Part model, mm, in its own coordinate system. A direction names the side the tool comes from. Round coordinates to 2 decimals unless told otherwise and drop trailing zeros. Order: outer loops, then holes, each group sorted by start corner. A loop starts at its lowest first (then second) coordinate and runs counter-clockwise, first axis right, second up. Notation, with made-up numbers: (73.25, 78.5) - (94.25, 78.5) arc R30 cw to (94.25, 101.5) - close; hole circle Ø7 at (87, 58.5). An arc over 180 degrees is marked (long way). Answer as a JSON object with one key per item and string values.
```python
from build123d import *

# Parameters (mm, degrees)
ESBO_O1_W                = 20
ESBO_O1_H                = 20
RESSALTO_EXTRUS_O1_DEPTH = 20
ESBO_O2_R                = 5
RESSALTO_EXTRUS_O2_DEPTH = 12
ESBO_O3_R                = 5
RESSALTO_EXTRUS_O3_DEPTH = 12
RESSALTO_EXTRUS_O4_START = 12
ESBO_O4_R                = 5
RESSALTO_EXTRUS_O4_DEPTH = 12
RESSALTO_EXTRUS_O5_START = 12
ESBO_O5_R                = 5
RESSALTO_EXTRUS_O5_DEPTH = 12
ESBO_O6_R                = 5
RESSALTO_EXTRUS_O6_DEPTH = 12
RESSALTO_EXTRUS_O7_START = 12
ESBO_O7_R                = 5
RESSALTO_EXTRUS_O7_DEPTH = 12


with BuildPart() as part:
    # Esboço1 → Ressalto-extrusão1 (new body)
    with BuildSketch(Plane.XY):
        Rectangle(ESBO_O1_W, ESBO_O1_H)
    extrude(amount=RESSALTO_EXTRUS_O1_DEPTH)

    # Esboço2 → Ressalto-extrusão2 (add)
    with BuildSketch(Plane(origin=(10, 0, 0), x_dir=(0, 0, -1), z_dir=(1, 0, 0))):
        with Locations((-10, 0)):
            Circle(ESBO_O2_R)
    extrude(amount=RESSALTO_EXTRUS_O2_DEPTH)

    # Esboço3 → Ressalto-extrusão3 (add)
    with BuildSketch(Plane(origin=(0, 10, 0), x_dir=(1, 0, 0), z_dir=(0, 1, 0))):
        with Locations(Location((0, -10, 0), (0, 0, 270))):
            Circle(ESBO_O3_R)
    extrude(amount=RESSALTO_EXTRUS_O3_DEPTH)

    # Esboço4 → Ressalto-extrusão4 (add)
    with BuildSketch(Plane.ZY.offset(10).offset(RESSALTO_EXTRUS_O4_START)):
        with Locations(Location((10, 0, 0), (0, 0, 180))):
            Circle(ESBO_O4_R)
    extrude(amount=-RESSALTO_EXTRUS_O4_DEPTH)

    # Esboço5 → Ressalto-extrusão5 (add)
    with BuildSketch(Plane.XZ.offset(10).offset(RESSALTO_EXTRUS_O5_START)):
        with Locations(Location((0, 10, 0), (0, 0, 90))):
            Circle(ESBO_O5_R)
    extrude(amount=-RESSALTO_EXTRUS_O5_DEPTH)

    # Esboço6 → Ressalto-extrusão6 (add)
    with BuildSketch(Plane(origin=(0, 0, 0), x_dir=(-1, 0, 0), z_dir=(0, 0, -1))):
        Circle(ESBO_O6_R)
    extrude(amount=RESSALTO_EXTRUS_O6_DEPTH)

    # Esboço7 → Ressalto-extrusão7 (add)
    with BuildSketch(Plane.XY.offset(20).offset(RESSALTO_EXTRUS_O7_START)):
        with Locations(Location((0, 0, 0), (0, 0, 180))):
            Circle(ESBO_O7_R)
    extrude(amount=-RESSALTO_EXTRUS_O7_DEPTH)


solid = part.part
```
Item 1: Drop flat-ended pins along their axis: P1, Ø3, axis at x = 8, z = 4.5, coming from the -Y side; P2, Ø1, axis at y = 3, z = 27, coming from the +X side; P3, Ø2, axis at y = -5, z = -1.5, coming from the +X side. Give the stop position or say it passes through.
Taken from the geometry:
{"P1": "y = -10", "P2": "x = 4.33", "P3": "x = 3"}
Item 2: Cut at D-D (y = -15). Write the cut outline in (x, z), plus the area to 3 significant figures.
Taken from the geometry:
{"outline": "circle Ø10 at (0, 10)", "area": "78.5 mm2"}
Item 3: Cut at A-A (z = 10). Write the cut outline in (x, y).
Taken from the geometry:
{"outline": "(-22, -5) - (-10, -5) - (-10, -10) - (-5, -10) - (-5, -22) - (5, -22) - (5, -10) - (10, -10) - (10, -5) - (22, -5) - (22, 5) - (10, 5) - (10, 10) - (5, 10) - (5, 22) - (-5, 22) - (-5, 10) - (-10, 10) - (-10, 5) - (-22, 5) - close"}
Item 4: Cut at B-B (y = 0). Write the cut outline in (x, z), plus the area to 3 significant figures.
Taken from the geometry:
{"outline": "(-22, 5) - (-10, 5) - (-10, 0) - (-5, 0) - (-5, -12) - (5, -12) - (5, 0) - (10, 0) - (10, 5) - (22, 5) - (22, 15) - (10, 15) - (10, 20) - (5, 20) - (5, 32) - (-5, 32) - (-5, 20) - (-10, 20) - (-10, 15) - (-22, 15) - close", "area": "880 mm2"}
Item 5: Probe L1, parallel to Z at x = -1, y = 7; L2, parallel to Y at x = -6, z = 10. List the from-to ranges inside material, lowest first. Write a range as from..to.
Taken from the geometry:
{"L1": "0..20", "L2": "-10..10"}
Item 6: Cut at C-C (x = -7). Write the cut outline in (y, z), plus the area to 3 significant figures.
Taken from the geometry:
{"outline": "(-10, 0) - (10, 0) - (10, 20) - (-10, 20) - close", "area": "400 mm2"}
Item 7: Tool access for faces 1 (the flat face through (10, -2, 5)), 2 (the flat face through (-2, -10, 5)), 3 (the cylindrical face through (1.08, -4.88, -5.92)): list every direction of +Z, -Z, +X, -X, +Y, -Y with a clear straight run to the whole face (end or side of a thin tool).
Taken from the geometry:
{"face 1": "+X", "face 2": "-Y", "face 3": "-Z"}
